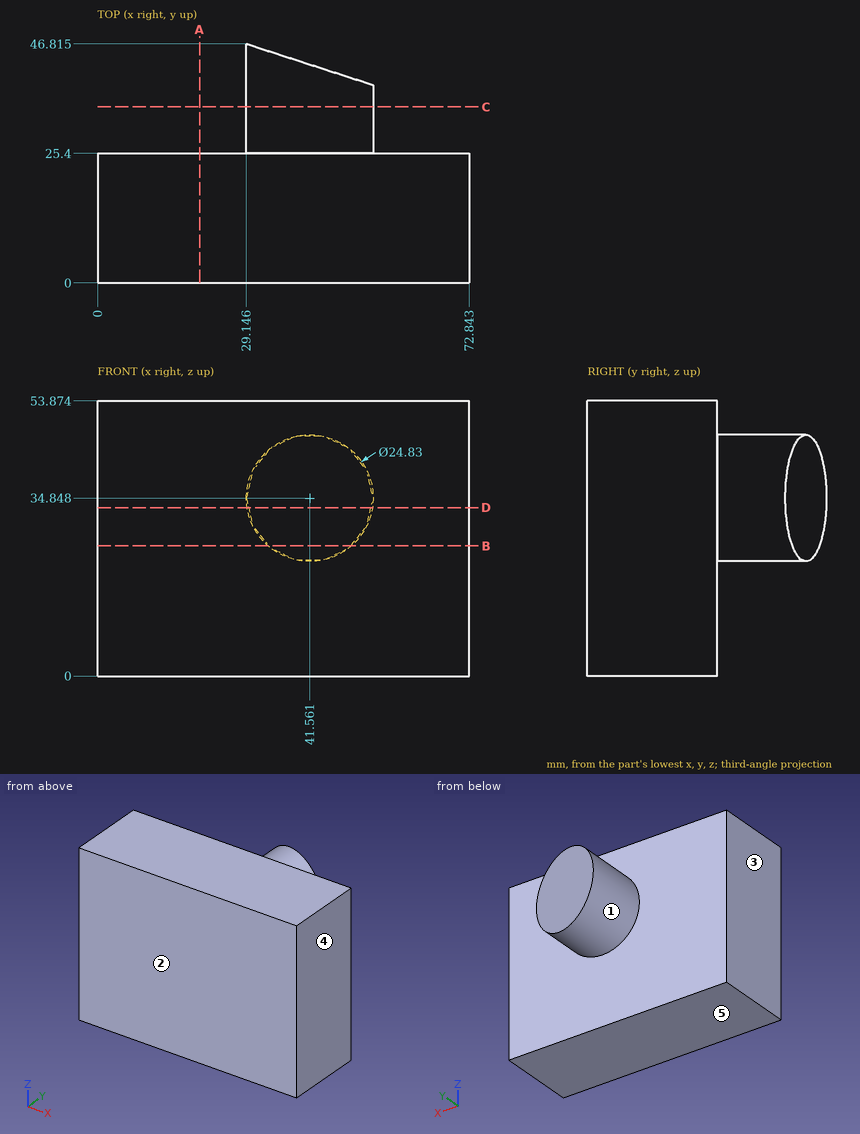
Input: dimensioned drawing with shaded views. Units: mm. Origin: part minimum x, y, z. A direction names the side the tool comes from. Round coordinates to 2 decimals unless told otherwise and drop trailing zeros. Loops run counter-clockwise (first coordinate to the right, second up) from the corner with the lowest first, then second, coordinate; pieces in that order, holes last. Notation, with made-up numbers: M 35,-4.75 L 72,-4.75 A18 cw 72,8.25 Z; hole C 19.5,-13.5 d3. An arc over 180 degrees is marked long. Return JSON: item names as keys, results as strings. Group by question number.
1. Section query D-D on z = 33. Output: boundary loops of the cut face in (x, y).
2. Mould query, pull axis X, two halves, no side actions, for the marked faces 3, 4 and 5. Classes: released by +X, released by -X, zero draft, split by the parting line, or undercut.
3. Pin query (flat end, axial travel): pin 1 (4 mm diameter, centred on y = 32.5, z = 28.5, fed in from +X); pin 2 (5 mm diameter, centred on y = 25.5, z = 42.5, fed in from -X); pin 3 (8 mm diameter, centred on x = 41, y = 38, fed in from +Z); pin 4 (1 mm diameter, centred on y = 35.5, z = 41, fed in from +X) (1 decimal). Return the tip coordinate at first contact, or that it passes through.
4. Reachability of the marked faces 1 and 2 from +Z, -Z, +X, -X, +Y, -Y: full face, straight path, thin tool, end or side. Return the list, or none.
5. Material intervals for line 1 along Y through (x, z) = (13.5, 24.5); line 2 along Z through (x, y) = (35.5, 39) (1 decimal), sorted ascending. Write a range as from..to.
6. Section query A-A on x = 20. Output: boundary loops of the cut face in (y, z) (1 decimal), and give its area (3 significant figures).
7. Section query B-B on z = 25.5. Output: boundary loops of the cut face in (x, y) (1 decimal), and give its area (3 significant figures).
8. Section query C-C on y = 34.5. Output: boundary loops of the cut face in (x, z) (1 decimal).
Checks:
{
 "1": {"outline": "M 0,0 L 72.84,0 L 72.84,25.4 L 53.84,25.4 L 53.84,38.8 L 29.28,46.77 L 29.28,25.4 L 0,25.4 Z"},
 "2": {"face 3": "released by -X", "face 4": "released by +X", "face 5": "zero draft"},
 "3": {"pin 1": "stops at x = 53.19", "pin 2": "stops at x = 0", "pin 3": "stops at z = 47.26", "pin 4": "stops at x = 52.6"},
 "4": {"face 1": "+Y", "face 2": "+Z, -Z, +X, -X, -Y"},
 "5": {"line 1": "y = 0..25.4", "line 2": "z = 24..45.7"},
 "6": {"outline": "M 0,0 L 25.4,0 L 25.4,53.9 L 0,53.9 Z", "area": "1,370 mm²"},
 "7": {"outline": "M 0,0 L 72.8,0 L 72.8,25.4 L 49.7,25.4 L 49.7,40.1 L 33.4,45.4 L 33.4,25.4 L 0,25.4 Z", "area": "2,130 mm²"},
 "8": {"outline": "C 41.6,34.8 d24.8"}
}
